Check sheet for the modelled part. Datum: model origin and axes. Units: mm. A direction names the side the tool comes from. Round coordinates to 2 decimals unless told otherwise and drop trailing zeros. Write each loop counter-clockwise with the first axis right and the second up, starting at its lowest first coordinate (ties: lowest second). Pieces come first, ordered by that corner, then holes.
Item 1: Depth check by flat-ended pin: pin 1 (1.5 mm diameter, centred on x = -5.5, z = 17.5, fed in from +Y); pin 2 (5.5 mm diameter, centred on x = -1, z = 35.5, fed in from +Y); pin 3 (6 mm diameter, centred on x = -23, y = 15, fed in from +Z). Enter the tip coordinate at first touch or a pass-through.
Item 2: Section check C-C, the plane x = 27. Record the cut outline in (y, z), plus the area to 3 significant figures.
Item 3: Set-up check for faces 4 (the flat face through (0, -5, 32)), 5 (the flat face through (22, 19, 2)), 6 (the cylindrical face through (25.302, 0.097, 0.986)), 7 (the flat face through (-2.5, 0, 32)): record each of +Z, -Z, +X, -X, +Y, -Y from which the full face is reachable in a straight line by a thin tool's end or side.
Item 4: Release check for a two-part mould opening along X. For faces 1 (the flat face through (0, 0, 40.5)), 2 (the cylindrical face through (-2.799, 21.317, 11.423)), 3 (the cylindrical face through (3.53, 28.61, 3.97)) record: pulls with the +X half, pulls with the -X half, needs draft (parallel to the pull), parting line crosses it, or undercut.
Item 5: Section check B-B, the plane y = -27.5. Record the cut outline in (x, z).
Item 6: Material ranges on line 1 along Y through (x, z) = (0, 4.65); line 2 along Y through (x, z) = (0, 1); line 3 along X through (y, z) = (1, 18.5), recorded low to high.
Item 7: Section check A-A, the plane x = 0. State how many separate pieces and enclosed holes the cut face has, plus the area to 3 significant figures.
from build123d import *

# Parameters (mm, degrees)
SKETCH1_R           = 35
SKETCH1_R_2         = 2.2
BOSS_EXTRUDE1_DEPTH = 2
SKETCH2_R           = 35
SKETCH2_R_2         = 3.7
BOSS_EXTRUDE2_DEPTH = 4
SKETCH4_R           = 20
BOSS_EXTRUDE3_DEPTH = 18.5
SKETCH6_W           = 5
SKETCH6_H           = 10
BOSS_EXTRUDE4_DEPTH = 16
SKETCH7_R           = 21.5
BOSS_EXTRUDE5_DEPTH = 11
SKETCH5_R           = 1.5
CUT_EXTRUDE1_DEPTH  = 25.5
CHAMFER1_SIZE       = 1


with BuildPart() as part:
    # Sketch1 → Boss-Extrude1 (new body)
    with BuildSketch(Plane.XY):
        Circle(SKETCH1_R)
        with Locations((0, 27.5)):
            Circle(SKETCH1_R_2, mode=Mode.SUBTRACT)
        with Locations((19.445436483, 19.445436483)):
            Circle(SKETCH1_R_2, mode=Mode.SUBTRACT)
        with Locations((27.5, 0)):
            Circle(SKETCH1_R_2, mode=Mode.SUBTRACT)
        with Locations((19.445436483, -19.445436483)):
            Circle(SKETCH1_R_2, mode=Mode.SUBTRACT)
        with Locations((0, -27.5)):
            Circle(SKETCH1_R_2, mode=Mode.SUBTRACT)
        with Locations((-19.445436483, -19.445436483)):
            Circle(SKETCH1_R_2, mode=Mode.SUBTRACT)
        with Locations((-27.5, 0)):
            Circle(SKETCH1_R_2, mode=Mode.SUBTRACT)
        with Locations((-19.445436483, 19.445436483)):
            Circle(SKETCH1_R_2, mode=Mode.SUBTRACT)
    extrude(amount=BOSS_EXTRUDE1_DEPTH)

    # Sketch2 → Boss-Extrude2 (add)
    with BuildSketch(Plane.XY.offset(2)):
        Circle(SKETCH2_R)
        with Locations((-27.5, 0)):
            Circle(SKETCH2_R_2, mode=Mode.SUBTRACT)
        with Locations((0, -27.5)):
            Circle(SKETCH2_R_2, mode=Mode.SUBTRACT)
        with Locations((27.5, 0)):
            Circle(SKETCH2_R_2, mode=Mode.SUBTRACT)
        with Locations((0, 27.5)):
            Circle(SKETCH2_R_2, mode=Mode.SUBTRACT)
        with Locations((19.445436483, 19.445436483)):
            Circle(SKETCH2_R_2, mode=Mode.SUBTRACT)
        with Locations((19.445436483, -19.445436483)):
            Circle(SKETCH2_R_2, mode=Mode.SUBTRACT)
        with Locations((-19.445436483, -19.445436483)):
            Circle(SKETCH2_R_2, mode=Mode.SUBTRACT)
        with Locations((-19.445436483, 19.445436483)):
            Circle(SKETCH2_R_2, mode=Mode.SUBTRACT)
    extrude(amount=BOSS_EXTRUDE2_DEPTH)

    # Sketch4 → Boss-Extrude3 (add)
    with BuildSketch(Plane.XY.offset(6)):
        Circle(SKETCH4_R)
    extrude(amount=BOSS_EXTRUDE3_DEPTH)

    # Sketch6 → Boss-Extrude4 (add)
    with BuildSketch(Plane.XY.offset(24.5)):
        Rectangle(SKETCH6_W, SKETCH6_H)
    extrude(amount=BOSS_EXTRUDE4_DEPTH)

    # Sketch7 → Boss-Extrude5 (add)
    with BuildSketch(Plane.XY.offset(6)):
        Circle(SKETCH7_R)
    extrude(amount=BOSS_EXTRUDE5_DEPTH)

    # Sketch5 → Cut-Extrude1 (cut, through all)
    with BuildSketch(Plane.XY.offset(24.5)):
        with Locations((-6, 0)):
            Circle(SKETCH5_R)
        with Locations((6, 0)):
            Circle(SKETCH5_R)
    extrude(amount=-CUT_EXTRUDE1_DEPTH, mode=Mode.SUBTRACT)

    # Chamfer1
    chamfer1_edges = [part.edges().sort_by_distance(p)[0] for p in [
        (-20, 0, 24.5),
    ]]
    chamfer(chamfer1_edges, length=CHAMFER1_SIZE)


solid = part.part
Values found:
1. pin 1: stops at y = 20.92
1. pin 2: stops at y = 5
1. pin 3: stops at z = 6
2. outline: (-22.27, 0) - (-2.14, 0) - (-2.14, 2) - (-3.67, 2) - (-3.67, 6) - (-22.27, 6) - close; (2.14, 0) - (22.27, 0) - (22.27, 6) - (3.67, 6) - (3.67, 2) - (2.14, 2) - close
2. area: 229 mm2
3. face 4: +Z, +X, -X, -Y
3. face 5: +Z
3. face 6: +Z, -Z
3. face 7: +Z, -X, +Y, -Y
4. face 1: needs draft
4. face 2: parting line crosses it
4. face 3: undercut
5. outline: (-21.65, 0) - (-2.2, 0) - (-2.2, 2) - (-3.7, 2) - (-3.7, 6) - (-21.65, 6) - close; (2.2, 0) - (21.65, 0) - (21.65, 6) - (3.7, 6) - (3.7, 2) - (2.2, 2) - close
6. line 1: y = -35 to -31.2, -23.8 to 23.8, 31.2 to 35
6. line 2: y = -35 to -29.7, -25.3 to 25.3, 29.7 to 35
6. line 3: x = -19.97 to -7.12, -4.88 to 4.88, 7.12 to 19.97
7. separate pieces: 3
7. enclosed holes: 0
7. area: 1,280 mm2
